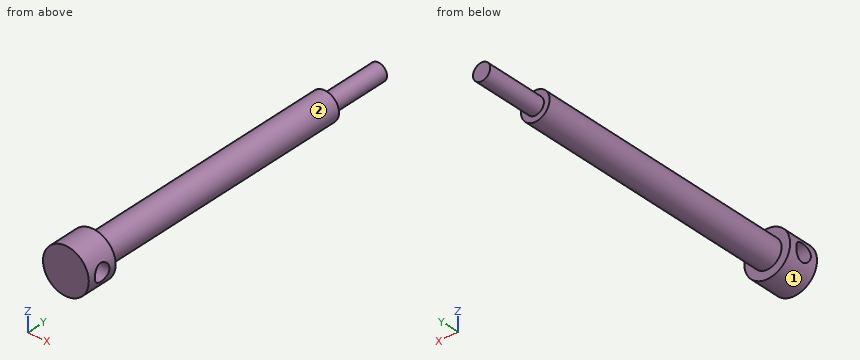
from build123d import *

# Parameters (mm, degrees)
SCHIZZO1_R                    = 8
ESTRUSIONE_ESTRUSIONE1_DEPTH  = 128
TAGLIO_ESTRUSIONE1_START      = -22
SCHIZZO2_R                    = 8
SCHIZZO2_R_2                  = 3
TAGLIO_ESTRUSIONE1_DEPTH      = 22
TAGLIO_ESTRUSIONE2_START      = -95
SCHIZZO5_R                    = 8
SCHIZZO5_R_2                  = 5
TAGLIO_ESTRUSIONE2_DEPTH      = 95
TAGLIO_ESTRUSIONE3_DEPTH      = 129.499027234
TAGLIO_ESTRUSIONE3_DEPTH_BACK = 129.499027234
SCHIZZO9_R                    = 3


with BuildPart() as part:
    # Schizzo1 → Estrusione-Estrusione1 (new body)
    with BuildSketch(Plane(origin=(0, 0, 0), x_dir=(1, 0, 0), z_dir=(0, 1, 0))):
        with Locations(Location((0, 0, 0), (0, 0, 270))):
            Circle(SCHIZZO1_R)
    extrude(amount=ESTRUSIONE_ESTRUSIONE1_DEPTH)

    # Schizzo2 → Taglio-Estrusione1 (cut)
    with BuildSketch(Plane(origin=(0, 128, 0), x_dir=(1, 0, 0), z_dir=(0, 1, 0)).offset(TAGLIO_ESTRUSIONE1_START)):
        with Locations(Location((0, 0, 0), (0, 0, 270))):
            Circle(SCHIZZO2_R)
        with Locations(Location((0, 0, 0), (0, 0, 270))):
            Circle(SCHIZZO2_R_2, mode=Mode.SUBTRACT)
    extrude(amount=TAGLIO_ESTRUSIONE1_DEPTH, mode=Mode.SUBTRACT)

    # Schizzo5 → Taglio-Estrusione2 (cut)
    with BuildSketch(Plane(origin=(0, 106, 0), x_dir=(1, 0, 0), z_dir=(0, 1, 0)).offset(TAGLIO_ESTRUSIONE2_START)):
        with Locations(Location((0, 0, 0), (0, 0, 270))):
            Circle(SCHIZZO5_R)
        with Locations(Location((0, 0, 0), (0, 0, 270))):
            Circle(SCHIZZO5_R_2, mode=Mode.SUBTRACT)
    extrude(amount=TAGLIO_ESTRUSIONE2_DEPTH, mode=Mode.SUBTRACT)

    # Schizzo9 → Taglio-Estrusione3 (cut, two sides: drawn at the far end of the back side and taken through both)
    with BuildSketch(Plane(origin=(0, 0, 0), x_dir=(0, 0, -1), z_dir=(1, 0, 0)).offset(-TAGLIO_ESTRUSIONE3_DEPTH_BACK)):
        with Locations((0, 5.5)):
            Circle(SCHIZZO9_R)
    extrude(amount=TAGLIO_ESTRUSIONE3_DEPTH + TAGLIO_ESTRUSIONE3_DEPTH_BACK, mode=Mode.SUBTRACT)


solid = part.part
Verification items for the finished model (mm, model axes). Face numbers are marked on the shaded views. A direction names the side the tool comes from. Give positions to 0.01 mm unless a question says otherwise; leave off trailing zeros. Write each loop counter-clockwise with the first axis right and the second up, starting at its lowest first coordinate (ties: lowest second). Pieces come first, ordered by that corner, then holes. Notation, with made-up numbers: M 30.25,-7.75 L 55.25,-7.75 A21 ccw 55.25,1.25 Z; hole C -33,63 d6. An arc over 180 degrees is marked long. Put each result on its own line as item: value. Start each with the question number.
1. Section check B-B (x = 0). Record the cut outline in (y, z), and give its area (3 significant figures).
2. Section check C-C (y = 5.5). Record the cut outline in (x, z).
3. Section check D-D (y = 78). Record the cut outline in (x, z), and give its area (3 significant figures).
4. Section check A-A (z = 0). Record the cut outline in (x, y).
5. Set-up check for the marked faces 1 and 2: record each of +Z, -Z, +X, -X, +Y, -Y from which the full face is reachable in a straight line by a thin tool's end or side.
6. Go/stop test with flat-tipped pins: pin 1 Ø5 at (y, z) = (5.5, 0) entering from -X; pin 2 Ø5 at (x, y) = (0.5, 24) entering from -Z; pin 3 Ø1.5 at (x, z) = (5.5, -5.5) entering from +Y; pin 4 Ø1.5 at (x, y) = (-4.5, 100) entering from -Z. Record where each tip stops, or that it passes through.
7. Scan lines: line 1 along Y through (x, z) = (-1.25, 0); line 2 along Y through (x, z) = (4.25, 5.25); line 3 along Y through (x, z) = (1.5, -2.5). Record each from-to range of solid material in increasing order. Write a range as [from, to].
Answer list:
1. outline: M 0,-8 L 11,-8 L 11,-5 L 106,-5 L 106,-3 L 128,-3 L 128,3 L 106,3 L 106,5 L 11,5 L 11,8 L 0,8 Z; hole C 5.5,0 d6
1. area: 1,230 mm2
2. outline: M -7.42,-3 A8 ccw 7.42,-3 Z; M -7.42,3 L 7.42,3 A8 ccw Z
3. outline: C 0,0 d10
3. area: 78.5 mm2
4. outline: M -8,0 L 8,0 L 8,2.5 L -8,2.5 Z; M -8,8.5 L 8,8.5 L 8,11 L 5,11 L 5,106 L 3,106 L 3,128 L -3,128 L -3,106 L -5,106 L -5,11 L -8,11 Z
5. face 1: +Y, -Y
5. face 2: +Y
6. pin 1: through
6. pin 2: z = -5
6. pin 3: y = 11
6. pin 4: z = -3.31
7. line 1: [0, 2.5], [8.5, 128]
7. line 2: [0, 11]
7. line 3: [0, 3.84], [7.16, 128]
